Could you check a few things on this model? Use its own coordinates, in mm. A direction names the side the tool comes from. Coordinates: 2 decimals unless noted, no trailing zeros. Loops run counter-clockwise (first coordinate to the right, second up) from the corner with the lowest first, then second, coordinate; pieces in that order, holes last. Notation, with made-up numbers: (-32, -40) - (-3, -40) arc R17 ccw to (-3, -36) - close; hole circle Ø1 at (60, -12.5). An arc over 180 degrees is marked (long way). One line per item, written item: value. Start each with the question number.
(1) If we section it at D-D on z = 2.5: Write out the boundary of the cut face in (x, y).
(2) On a 3-axis mill with a long thin cutter (end or side, diameter ignored), from which of +Z, -Z, +X, -X, +Y, -Y can I reach the whole of each face in a straight line? I mean faces 1 (the face through (0, 2, -20)), 2 (the face through (-3.817, 7.465, 17.465)), 3 (the face through (0, 7, 15)). Say none if no direction works.
(3) If we section it at C-C on z = -5: Write out the boundary of the cut face in (x, y), then the cut area to 3 significant figures.
(4) I'm going to push flat-ended pins straight in: P1, Ø1.5, axis at x = -0.5, y = 8.5, coming from the -Z side; P2, Ø12, axis at x = 0, z = -8, coming from the +Y side. Where does each tip first touch, or does it pass through?
(5) If we section it at B-B on y = 3.25: Write out the boundary of the cut face in (x, z), then the cut area to 3 significant figures.
(6) If we mould it in two halves opening along X, with no side actions, what happens to faces 4 (the face through (30, 3, 15)), 5 (the face through (0, 0, 0)), 6 (the face through (9.1, 2.5, -6.2))? For each: pulls with the +X half, pulls with the -X half, needs draft (parallel to the pull), parting line crosses it, or undercut.
(7) If we section it at A-A on x = -10: Write out the boundary of the cut face in (y, z).
(8) If I drill on line 1 along X through (y, z) = (2.8, -5); line 2 along Y through (x, z) = (-3.5, 2.5); line 3 along X through (y, z) = (9.25, 17), over which ranges is the centre line in solid material (lowest first)? Write a range as from..to.
```python
from build123d import *

# Parameters (mm, degrees)
SKETCH1_W           = 70
SKETCH1_H           = 40
BOSS_EXTRUDE1_DEPTH = 5
SKETCH2_R           = 1.5
CUT_EXTRUDE1_DEPTH  = 5
SKETCH2_3_R         = 1.5
CUT_EXTRUDE2_DEPTH  = 5
SKETCH3_R           = 1.5
BOSS_EXTRUDE2_DEPTH = 5
SKETCH3_3_R         = 1.5
BOSS_EXTRUDE3_DEPTH = 5
CUT_EXTRUDE3_DEPTH  = 10
CUT_EXTRUDE4_DEPTH  = 10
BOSS_EXTRUDE4_DEPTH = 5


with BuildPart() as part:
    # Sketch1 → Boss-Extrude1 (new body)
    with BuildSketch(Plane(origin=(0, 0, 0), x_dir=(1, 0, 0), z_dir=(0, 1, 0))):
        Rectangle(SKETCH1_W, SKETCH1_H)
    extrude(amount=BOSS_EXTRUDE1_DEPTH)

    # Sketch2 → Cut-Extrude1 (cut)
    with BuildSketch(Plane(origin=(0, 5, 0), x_dir=(1, 0, 0), z_dir=(0, 1, 0))):
        with Locations(Location((-10, 5, 0), (0, 0, 270))):
            Circle(SKETCH2_R)
    extrude(amount=-CUT_EXTRUDE1_DEPTH, mode=Mode.SUBTRACT)

    # Sketch2_3 → Cut-Extrude2 (cut)
    with BuildSketch(Plane(origin=(0, 5, 0), x_dir=(1, 0, 0), z_dir=(0, 1, 0))):
        with Locations(Location((-10, 5, 0), (0, 0, 270))):
            Circle(SKETCH2_3_R)
        with Locations(Location((10, 5, 0), (0, 0, 270))):
            Circle(SKETCH2_3_R)
    extrude(amount=-CUT_EXTRUDE2_DEPTH, mode=Mode.SUBTRACT)

    # Sketch3 → Boss-Extrude2 (add)
    with BuildSketch(Plane(origin=(0, 5, 0), x_dir=(1, 0, 0), z_dir=(0, 1, 0))):
        with Locations(Location((-5, -15, 0), (0, 0, 270))):
            Circle(SKETCH3_R)
    extrude(amount=BOSS_EXTRUDE2_DEPTH)

    # Sketch3_3 → Boss-Extrude3 (add)
    with BuildSketch(Plane(origin=(0, 5, 0), x_dir=(1, 0, 0), z_dir=(0, 1, 0))):
        with Locations(Location((-5, -15, 0), (0, 0, 270))):
            Circle(SKETCH3_3_R)
        with Locations(Location((5, -15, 0), (0, 0, 270))):
            Circle(SKETCH3_3_R)
    extrude(amount=BOSS_EXTRUDE3_DEPTH)

    # Sketch8 → Cut-Extrude3 (cut)
    with BuildSketch(Plane(origin=(0, 5, 0), x_dir=(1, 0, 0), z_dir=(0, 1, 0))):
        Polygon((-25, -20), (-35, -10), (-35, -20), align=None)
    extrude(amount=-CUT_EXTRUDE3_DEPTH, mode=Mode.SUBTRACT)

    # Sketch9 → Cut-Extrude4 (cut)
    with BuildSketch(Plane(origin=(0, 5, 0), x_dir=(1, 0, 0), z_dir=(0, 1, 0))):
        Polygon((35, -20), (25, -20), (35, -10), align=None)
    extrude(amount=-CUT_EXTRUDE4_DEPTH, mode=Mode.SUBTRACT)

    # Sketch13 → Boss-Extrude4 (add)
    with BuildSketch(Plane(origin=(0, 5, 0), x_dir=(1, 0, 0), z_dir=(0, 1, 0))):
        Polygon((-6.2, -20), (6.2, -20), (1.5, -15), (-1.5, -15), align=None)
    extrude(amount=BOSS_EXTRUDE4_DEPTH)


solid = part.part
```
Values:
1. outline: (-35, 0) - (35, 0) - (35, 5) - (-35, 5) - close
2. face 1: -Z, +X, -X, +Y, -Y
2. face 2: +Y
2. face 3: -Z, +Y
3. outline: (-35, 0) - (-11.5, 0) - (-11.5, 5) - (-35, 5) - close; (-8.5, 0) - (8.5, 0) - (8.5, 5) - (-8.5, 5) - close; (11.5, 0) - (35, 0) - (35, 5) - (11.5, 5) - close
3. area: 320 mm2
4. P1: stops at z = 15
4. P2: stops at y = 5
5. outline: (-35, -20) - (35, -20) - (35, 10) - (25, 20) - (-25, 20) - (-35, 10) - close; hole circle Ø3 at (-10, -5); hole circle Ø3 at (10, -5)
5. area: 2,690 mm2
6. face 4: pulls with the +X half
6. face 5: needs draft
6. face 6: undercut
7. outline: (0, -20) - (5, -20) - (5, -6.5) - (0, -6.5) - close; (0, -3.5) - (5, -3.5) - (5, 20) - (0, 20) - close
8. line 1: x = -35..-11.5, -8.5..8.5, 11.5..35
8. line 2: y = 0..5
8. line 3: x = -3.38..3.38
